from build123d import *

# Parameters (mm, degrees)
BOSS_EXTRUDE1_DEPTH = 30
SKETCH3_R           = 7.75
CUT_EXTRUDE1_DEPTH  = 30
FILLET1_R           = 5
SKETCH4_W           = 36
SKETCH4_H           = 30
BOSS_EXTRUDE2_DEPTH = 4


with BuildPart() as part:
    # Sketch2 → Boss-Extrude1 (new body)
    with BuildSketch(Plane(origin=(0, 0, 0), x_dir=(1, 0, 0), z_dir=(0, 1, 0))):
        Polygon((-14.863905325, 0), (-6.863905325, 0), (-6.863905325, 20), (13.136094675, 20), (13.136094675, 0), (21.136094675, 0), (21.136094675, -3), (-14.863905325, -3), align=None)
    extrude(amount=BOSS_EXTRUDE1_DEPTH)

    # Sketch3 → Cut-Extrude1 (cut)
    with BuildSketch(Plane.XZ):
        with Locations(Location((3.136094675, -8.5, 0), (0, 0, 270))):
            Circle(SKETCH3_R)
    extrude(amount=-CUT_EXTRUDE1_DEPTH, mode=Mode.SUBTRACT)

    # Fillet1
    fillet1_edges = [part.edges().sort_by_distance(p)[0] for p in [
        (-6.863905325, 15, -20),
        (13.136094675, 15, -20),
    ]]
    fillet(fillet1_edges, radius=FILLET1_R)

    # Sketch4 → Boss-Extrude2 (add)
    with BuildSketch(Plane.XY.offset(3)):
        with Locations((3.136094675, 15)):
            Rectangle(SKETCH4_W, SKETCH4_H)
    extrude(amount=BOSS_EXTRUDE2_DEPTH)


solid = part.part
The listing builds one solid part. Answer for the finished solid, in the listing's coordinates (mm). A direction names the side the tool comes from. Coordinates: 2 decimals unless noted, no trailing zeros. Loops run counter-clockwise (first coordinate to the right, second up) from the corner with the lowest first, then second, coordinate; pieces in that order, holes last. Notation, with made-up numbers: M 14.5,-39 L 62.5,-39 A28 ccw 62.5,-21 Z; hole C -33.5,22.25 d7. An arc over 180 degrees is marked long. Answer in a Markdown table with one row per item.
1) Find section B-B (x = 6). Determine the outline of the cut face in (y, z).
Answers below:
| item | result |
|---|---|
| outline | M 0,-20 L 30,-20 L 30,-15.7 L 0,-15.7 Z; M 0,-1.3 L 30,-1.3 L 30,7 L 0,7 Z |
2) Find section C-C (y = 13). Determine the outline of the cut face in (x, z), then the cut area to 3 significant figures.
Answers below:
| item | result |
|---|---|
| outline | M -14.86,0 L -6.86,0 L -6.86,-15 A5 ccw -1.86,-20 L 8.14,-20 A5 ccw 13.14,-15 L 13.14,0 L 21.14,0 L 21.14,7 L -14.86,7 Z; hole C 3.14,-8.5 d15.5 |
| area | 453 mm^2 |
3) Given pin 1 (1 mm diameter, centred on x = -3, y = 7.5, fed in from -Z); pin 2 (8 mm diameter, centred on x = 14, y = 23.5, fed in from -Z); pin 3 (2.5 mm diameter, centred on x = -12.5, y = 13.5, fed in from -Z), each flat-ended and moving along its own axis, determine where each tip first touches the part or whether it passes through.
Answers below:
| item | result |
|---|---|
| pin 1 | z = -19.96 |
| pin 2 | z = -19.64 |
| pin 3 | z = 0 |
4) Determine the mould class of faces 4 (the cylindrical face through (-1.58, 14.79, -2.35)), 5 (the flat face through (3, 15, 7)), 6 (the flat face through (21.136, 15, 3)), 7 (the flat face through (3, 15, -20)) for opening direction Z: released by +Z, released by -Z, zero draft, split by the parting line, or undercut.
Answers below:
| item | result |
|---|---|
| face 4 | undercut |
| face 5 | released by +Z |
| face 6 | zero draft |
| face 7 | released by -Z |
5) Find the intervals of material crossed by probe 1 along X at (y, z) = (10, -8.5); probe 2 along X at (y, z) = (5.5, -6.75); probe 3 along Z at (x, y) = (16, 2.75), in increasing order.
Answers below:
| item | result |
|---|---|
| probe 1 | -6.86 to -4.61, 10.89 to 13.14 |
| probe 2 | -6.86 to -4.41, 10.69 to 13.14 |
| probe 3 | 0 to 7 |
6) Find section A-A (z = -8.5). Determine the outline of the cut face in (x, y), then the cut area to 3 significant figures.
Answers below:
| item | result |
|---|---|
| outline | M -6.86,0 L -4.61,0 L -4.61,30 L -6.86,30 Z; M 10.89,0 L 13.14,0 L 13.14,30 L 10.89,30 Z |
| area | 135 mm^2 |
7) Find section D-D (x = 15). Determine the outline of the cut face in (y, z).
Answers below:
| item | result |
|---|---|
| outline | M 0,0 L 30,0 L 30,7 L 0,7 Z |
8) Which of the six approach directions +Z, -Z, +X, -X, +Y, -Y give full straight-line access (tool end or side, diameter ignored) to faces 1 (the flat face through (-11, 15, 0)), 2 (the flat face through (-1, 0, -1)), 3 (the flat face through (17, 15, 0))?
Answers below:
| item | result |
|---|---|
| face 1 | -Z, -X, +Y, -Y |
| face 2 | +Z, -Z, +X, -X, -Y |
| face 3 | -Z, +X, +Y, -Y |
